```python
from build123d import *

# Parameters (mm, degrees)
SKETCH1_W           = 10
SKETCH1_H           = 8
BOSS_EXTRUDE1_DEPTH = 1.5
SKETCH2_W           = 1.5
SKETCH2_H           = 8
BOSS_EXTRUDE2_DEPTH = 8
SKETCH4_R           = 1.25
CUT_EXTRUDE1_DEPTH  = 14.360389216
SKETCH5_R           = 1.2
CUT_EXTRUDE2_DEPTH  = 12.456439237


with BuildPart() as part:
    # Sketch1 → Boss-Extrude1 (new body)
    with BuildSketch(Plane(origin=(0, 0, 0), x_dir=(1, 0, 0), z_dir=(0, 1, 0))):
        Rectangle(SKETCH1_W, SKETCH1_H)
    extrude(amount=BOSS_EXTRUDE1_DEPTH)

    # Sketch2 → Boss-Extrude2 (add)
    with BuildSketch(Plane(origin=(0, 1.5, 0), x_dir=(1, 0, 0), z_dir=(0, 1, 0))):
        with Locations((-4.25, 0)):
            Rectangle(SKETCH2_W, SKETCH2_H)
    boss_extrude2 = extrude(amount=BOSS_EXTRUDE2_DEPTH)

    # Sketch4 → Cut-Extrude1 (cut, through all)
    with BuildSketch(Plane(origin=(-3.5, 0, 0), x_dir=(0, 0, -1), z_dir=(1, 0, 0))):
        with Locations((0, 5.5)):
            Circle(SKETCH4_R)
    cut_extrude1 = extrude(amount=-CUT_EXTRUDE1_DEPTH, mode=Mode.SUBTRACT)

    # Mirror2: Boss-Extrude2, Cut-Extrude1 across plane
    add(boss_extrude2.mirror(Plane(origin=(0, 0, 0), x_dir=(0, 0, 1), z_dir=(1, 0, 0))))
    add(cut_extrude1.mirror(Plane(origin=(0, 0, 0), x_dir=(0, 0, 1), z_dir=(1, 0, 0))), mode=Mode.SUBTRACT)

    # Sketch5 → Cut-Extrude2 (cut, through all)
    with BuildSketch(Plane(origin=(0, 0, 0), x_dir=(1, 0, 0), z_dir=(0, 1, 0))):
        with Locations(Location((0, 0, 0), (0, 0, 90))):
            Circle(SKETCH5_R)
    extrude(amount=CUT_EXTRUDE2_DEPTH, mode=Mode.SUBTRACT)


solid = part.part
```
The model under review builds one solid part; all positions refer to its coordinate system, in mm. A direction names the side the tool comes from. Round coordinates to 2 decimals unless told otherwise and drop trailing zeros. Loops run counter-clockwise (first coordinate to the right, second up) from the corner with the lowest first, then second, coordinate; pieces in that order, holes last. Notation, with made-up numbers: (15, -32.5) - (31, -32.5) arc R16 cw to (31, -24.5) - close; hole circle Ø10 at (81.5, 32). An arc over 180 degrees is marked (long way). Write each question's results on one line, items separated by ' | '. Start each with the question number.
Q1. Take a section at D-D on y = 5.5. Give the boundary of the cut face in (x, z), plus the area to 3 significant figures.
Q2. Wall thickness on line 1 along X through (y, z) = (2.5, 2.75); line 2 along Y through (x, z) = (4.3, 0); line 3 along X through (y, z) = (0.8, 0): over which ranges is each line inside the solid? List them lowest first. Write a range as [from, to].
Q3. Take a section at B-B on y = 2.25. Give the boundary of the cut face in (x, z), plus the area to 3 significant figures.
Q4. Draft analysis for pull direction X (two halves, no side actions). For faces 3 (the cylindrical face through (-1.01, 0.74, -0.65)), 4 (the flat face through (-5, 4, 0)), 5 (the cylindrical face through (4.24, 4.28, 0.27)), 6 (the flat face through (-3.5, 4, 0)), state which applies: pulls with the +X half, pulls with the -X half, needs draft (parallel to the pull), parting line crosses it, or undercut.
Q5. Take a section at A-A on x = 0. Give the boundary of the cut face in (y, z), plus the area to 3 significant figures.
Q6. Take a section at C-C on z = 0. Give the boundary of the cut face in (x, y).
Q7. Tool access review of faces 1 (the flat face through (0, 1, 4)), 2 (the flat face through (3.5, 4, 0)): name each direction out of +Z, -Z, +X, -X, +Y, -Y from which nothing blocks a thin tool from reaching the whole face with its end or side.
Data:
1) outline: (-5, -4) - (-3.5, -4) - (-3.5, -1.25) - (-5, -1.25) - close; (-5, 1.25) - (-3.5, 1.25) - (-3.5, 4) - (-5, 4) - close; (3.5, -4) - (5, -4) - (5, -1.25) - (3.5, -1.25) - close; (3.5, 1.25) - (5, 1.25) - (5, 4) - (3.5, 4) - close | area: 16.5 mm²
2) line 1: x = [-5, -3.5], [3.5, 5] | line 2: y = [0, 4.25], [6.75, 9.5] | line 3: x = [-5, -1.2], [1.2, 5]
3) outline: (-5, -4) - (-3.5, -4) - (-3.5, 4) - (-5, 4) - close; (3.5, -4) - (5, -4) - (5, 4) - (3.5, 4) - close | area: 24.0 mm²
4) face 3: undercut | face 4: pulls with the -X half | face 5: needs draft | face 6: undercut
5) outline: (0, -4) - (1.5, -4) - (1.5, -1.2) - (0, -1.2) - close; (0, 1.2) - (1.5, 1.2) - (1.5, 4) - (0, 4) - close | area: 8.40 mm²
6) outline: (-5, 0) - (-1.2, 0) - (-1.2, 1.5) - (-3.5, 1.5) - (-3.5, 4.25) - (-5, 4.25) - close; (-5, 6.75) - (-3.5, 6.75) - (-3.5, 9.5) - (-5, 9.5) - close; (1.2, 0) - (5, 0) - (5, 4.25) - (3.5, 4.25) - (3.5, 1.5) - (1.2, 1.5) - close; (3.5, 6.75) - (5, 6.75) - (5, 9.5) - (3.5, 9.5) - close
7) face 1: +Z, +X, -X, +Y, -Y | face 2: +Z, -Z, +Y
